Autodesk Inventor part; units mm, degrees
ref_plane "YZ Plane" through (0, 0, 0) normal (1, 0, 0) x (0, 1, 0)
ref_plane "XZ Plane" through (0, 0, 0) normal (0, 1, 0) x (-1, 0, 0)
ref_plane "XY Plane" through (0, 0, 0) normal (0, 0, 1) x (1, 0, 0)
sketch "Szkic1" plane through (0, 0, 0) normal (0, 0, 1) x (1, 0, 0)
  line L0 (-9.5177, 6.3249) -> (9.4823, 6.3249)
  line L1 (9.4823, 6.3249) -> (9.4823, -21.6751)
  line L2 (9.4823, -21.6751) -> (-9.5177, -21.6751)
  line L3 (-9.5177, -21.6751) -> (-9.5177, 6.3249)
  point P0 (0, 0)
  dimension "d0" = 19
  dimension "d1" = 28
extrude "Wyciągnięcie proste1" add sketch "Szkic1" along normal blind 12
chamfer "Faza1" distance 5 angle 45 2 edges at (9.4823, 6.3249, 6) (9.4823, -21.6751, 6)
fillet "Zaokrąglenie1" radius 4 2 edges at (-9.5177, 6.3249, 6) (-9.5177, -21.6751, 6)
sketch "Szkic2" plane through (0, 0, 0) normal (0, 0, -1) x (-1, 0, 0)
  line L0 (-4.4823, -21.6751) -> (5.5177, -21.6751)
  line L1 (5.5177, 6.3249) -> (-4.4823, 6.3249)
  arc A0 (5.5177, -21.6751) -> (9.5177, -17.6751) centre (5.5177, -17.6751) ccw
  line L2 (9.5177, -17.6751) -> (9.5177, 2.3249)
  arc A1 (9.5177, 2.3249) -> (5.5177, 6.3249) centre (5.5177, 2.3249) ccw
  line L3 (5.5177, 6.3249) -> (-4.4823, 6.3249)
  line L4 (-9.4823, 1.3249) -> (-4.4823, 6.3249)
  line L5 (-9.4823, 1.3249) -> (-9.4823, -16.6751)
  line L6 (-4.4823, -21.6751) -> (-9.4823, -16.6751)
  line L7 (-4.4823, -21.6751) -> (5.5177, -21.6751)
  line L8 (7.5177, 2.3249) -> (7.5177, -17.6751)
  arc A2 (5.5177, -19.6751) -> (7.5177, -17.6751) centre (5.5177, -17.6751) ccw
  line L9 (5.5177, -19.6751) -> (-3.6539, -19.6751)
  line L10 (-3.6539, -19.6751) -> (-7.4823, -15.8467)
  line L11 (-7.4823, -15.8467) -> (-7.4823, 0.4965)
  line L12 (-7.4823, 0.4965) -> (-3.6539, 4.3249)
  line L13 (-3.6539, 4.3249) -> (5.5177, 4.3249)
  arc A3 (7.5177, 2.3249) -> (5.5177, 4.3249) centre (5.5177, 2.3249) ccw
  line L14 (10.5177, 2.3249) -> (10.5177, -17.6751)
  line L15 (-10.4823, 2.3249) -> (-10.4823, -17.6751)
  circle A4 centre (0.5177, 11.8249) radius 2.5
  circle A5 centre (0.5177, -27.1751) radius 2.5
  line L16 (-10.4823, -17.6751) -> (-1.4174, -28.7579)
  line L17 (10.5177, 2.3249) -> (2.5396, 13.2953)
  line L18 (10.5177, -17.6751) -> (2.5396, -28.6455)
  line L19 (-10.4823, 2.3249) -> (-1.4174, 13.4077)
  point P0 (0, 0)
  dimension "d8" = 28
  dimension "d9" = 2
  dimension "d10" = 20
  dimension "d11" = 1
  dimension "d12" = 4
  dimension "d13" = 20
  dimension "d14" = 1
  dimension "d15" = 4
  dimension "d16" = 10
  dimension "d17" = 10
  dimension "d18" = 39
  dimension "d19" = 5.5
  dimension "d20" = 5
  dimension "d21" = 5
extrude "Wyciągnięcie proste2" add sketch "Szkic2" along normal blind 5.5 contours L6 L5 L4 L1 A1 L2 A0 L0 | L14 L18 A5 L16 L15 L19 A4 L17 | A4 | A5
extrude "Wyciągnięcie proste3" cut sketch "Szkic2" against normal blind 11 contours L8 A2 L9 L10 L11 L12 L13 A3
hole "Otwór1" at (-0.5177, 11.8249, 0) at (-0.5177, -27.1751, 0) direction (0, 0, -1) diameter 3 end through all
sketch "Szkic3" plane through (0, 0, -5.5) normal (0, 0, -1) x (-1, 0, 0)
  circle A0 centre (0.5177, 11.8249) radius 1.5
  circle A1 centre (0.5177, -27.1751) radius 1.5
  arc A2 (5.5177, -19.6751) -> (7.5177, -17.6751) centre (5.5177, -17.6751) ccw
  line L0 (5.5177, -19.6751) -> (-3.6539, -19.6751)
  line L1 (-3.6539, -19.6751) -> (-7.4823, -15.8467)
  line L2 (-7.4823, -15.8467) -> (-7.4823, 0.4965)
  line L3 (-7.4823, 0.4965) -> (-3.6539, 4.3249)
  line L4 (-3.6539, 4.3249) -> (5.5177, 4.3249)
  arc A3 (7.5177, 2.3249) -> (5.5177, 4.3249) centre (5.5177, 2.3249) ccw
  line L5 (7.5177, 2.3249) -> (7.5177, -17.6751)
  arc A4 (-1.4174, -28.7579) -> (2.5396, -28.6455) centre (0.5177, -27.1751) ccw
  line L6 (2.5396, -28.6455) -> (10.5177, -17.6751)
  line L7 (10.5177, -17.6751) -> (10.5177, 2.3249)
  line L8 (10.5177, 2.3249) -> (2.5396, 13.2953)
  arc A5 (2.5396, 13.2953) -> (-1.4174, 13.4077) centre (0.5177, 11.8249) ccw
  line L9 (-1.4174, 13.4077) -> (-10.4823, 2.3249)
  line L10 (-10.4823, 2.3249) -> (-10.4823, -17.6751)
  line L11 (-10.4823, -17.6751) -> (-1.4174, -28.7579)
  line L12 (6.5179, 7.8249) -> (-5.9837, 7.8249)
  line L13 (6.5179, -23.1751) -> (-5.9837, -23.1751)
  point P0 (0, 0)
  dimension "d33" = 31
  dimension "d34" = 39
  dimension "d35" = 4
extrude "Wyciągnięcie proste4" cut sketch "Szkic3" against normal blind 2 contours L11 L13 L6 A4 | L9 A5 L8 L12
fillet "Zaokrąglenie2" radius 1 4 edges at (-0.2671, 7.8249, -5.5) (-0.2671, 7.8249, -3.5) (-0.2671, -23.1751, -3.5) (-0.2671, -23.1751, -5.5)
fillet "Zaokrąglenie3" radius 5 4 edges at (-10.5177, 2.3249, -2.75) (-10.5177, -17.6751, -2.75) (10.4823, 2.3249, -2.75) (10.4823, -17.6751, -2.75)
sketch "Szkic4" plane through (0, 0, 11) normal (0, 0, -1) x (-1, 0, 0)
  line L0 (7.5177, 2.3249) -> (7.5177, -17.6751)
  arc A0 (7.5177, 2.3249) -> (5.5177, 4.3249) centre (5.5177, 2.3249) ccw
  line L1 (-3.6539, 4.3249) -> (5.5177, 4.3249)
  line L2 (-7.4823, 0.4965) -> (-3.6539, 4.3249)
  line L3 (-7.4823, -15.8467) -> (-7.4823, 0.4965)
  line L4 (-3.6539, -19.6751) -> (-7.4823, -15.8467)
  line L5 (5.5177, -19.6751) -> (-3.6539, -19.6751)
  arc A1 (5.5177, -19.6751) -> (7.5177, -17.6751) centre (5.5177, -17.6751) ccw
  line L6 (4.5177, 0.8249) -> (0.5177, 0.8249)
  line L7 (0.5177, 0.8249) -> (0.5177, -1.1751)
  line L8 (0.5177, -1.1751) -> (4.5177, -1.1751)
  line L9 (4.5177, -1.1751) -> (4.5177, 0.8249)
  line L10 (4.5177, -14.1751) -> (0.5177, -14.1751)
  line L11 (0.5177, -14.1751) -> (0.5177, -16.1751)
  line L12 (0.5177, -16.1751) -> (4.5177, -16.1751)
  line L13 (4.5177, -16.1751) -> (4.5177, -14.1751)
  line L14 (-1.4823, -6.6751) -> (-5.4823, -6.6751)
  line L15 (-5.4823, -6.6751) -> (-5.4823, -8.6751)
  line L16 (-5.4823, -8.6751) -> (-1.4823, -8.6751)
  line L17 (-1.4823, -8.6751) -> (-1.4823, -6.6751)
  point P0 (0, 0)
  dimension "d40" = 4
  dimension "d41" = 2
  dimension "d42" = 4
  dimension "d43" = 2
  dimension "d44" = 4
  dimension "d45" = 2
  dimension "d46" = 13
  dimension "d47" = 24
  dimension "d48" = 3.5
  dimension "d49" = 5.5
  dimension "d50" = 2
  dimension "d51" = 3
  dimension "d52" = 3
extrude "Wyciągnięcie proste5" add sketch "Szkic4" along normal blind 15 contours L9 L8 L7 L6 | L13 L12 L11 L10 | L17 L16 L15 L14
fillet "Zaokrąglenie4" radius 2 6 edges at (1.4823, -7.6751, -4) (5.4823, -7.6751, -4) (-0.5177, -0.1751, -4) (-4.5177, -0.1751, -4) (-0.5177, -15.1751, -4) (-4.5177, -15.1751, -4)
sketch "Szkic5" plane through (0, 0, 12) normal (0, 0, 1) x (1, 0, 0)
  arc A0 (-9.5177, -17.6751) -> (-5.5177, -21.6751) centre (-5.5177, -17.6751) ccw
  line L0 (-5.5177, -21.6751) -> (4.4823, -21.6751)
  line L1 (9.4823, -16.6751) -> (4.4823, -21.6751)
  line L2 (9.4823, -16.6751) -> (9.4823, 1.3249)
  line L3 (4.4823, 6.3249) -> (9.4823, 1.3249)
  line L4 (4.4823, 6.3249) -> (-5.5177, 6.3249)
  arc A1 (-5.5177, 6.3249) -> (-9.5177, 2.3249) centre (-5.5177, 2.3249) ccw
  line L5 (-9.5177, 2.3249) -> (-9.5177, -17.6751)
  line L6 (-0.5177, -14.1751) -> (-4.5177, -14.1751)
  line L7 (-4.5177, -16.1751) -> (-0.5177, -16.1751)
  line L8 (-4.5177, -14.1751) -> (-4.5177, -16.1751)
  line L9 (-0.5177, -16.1751) -> (-0.5177, -14.1751)
  line L10 (-4.5177, -1.1751) -> (-0.5177, -1.1751)
  line L11 (-0.5177, 0.8249) -> (-4.5177, 0.8249)
  line L12 (-4.5177, 0.8249) -> (-4.5177, -1.1751)
  line L13 (-0.5177, -1.1751) -> (-0.5177, 0.8249)
  line L14 (1.4823, -8.6751) -> (5.4823, -8.6751)
  line L15 (5.4823, -6.6751) -> (1.4823, -6.6751)
  line L16 (5.4823, -8.6751) -> (5.4823, -6.6751)
  line L17 (1.4823, -6.6751) -> (1.4823, -8.6751)
  line L18 (-5.5177, -17.1751) -> (0.4823, -17.1751)
  line L19 (0.4823, -17.1751) -> (0.4823, -13.1751)
  line L20 (0.4823, -13.1751) -> (-5.5177, -13.1751)
  line L21 (-5.5177, -13.1751) -> (-5.5177, -17.1751)
  line L22 (0.4823, -9.6751) -> (6.4823, -9.6751)
  line L23 (6.4823, -9.6751) -> (6.4823, -5.6751)
  line L24 (6.4823, -5.6751) -> (0.4823, -5.6751)
  line L25 (0.4823, -5.6751) -> (0.4823, -9.6751)
  line L26 (0.4823, 1.8249) -> (-5.5177, 1.8249)
  line L27 (-5.5177, 1.8249) -> (-5.5177, -2.1751)
  line L28 (-5.5177, -2.1751) -> (0.4823, -2.1751)
  line L29 (0.4823, -2.1751) -> (0.4823, 1.8249)
  point P0 (0, 0)
  dimension "d56" = 1
  dimension "d57" = 1
  dimension "d58" = 1
extrude "Wyciągnięcie proste6" add sketch "Szkic5" along normal blind 10 contours L9 L7 L8 L6 | L12 L11 L13 L10 | L17 L15 L16 L14
extrude "Wyciągnięcie proste7" add sketch "Szkic5" along normal blind 4 contours L21 L20 L19 L18 | L25 L24 L23 L22 | L29 L28 L27 L26
fillet "Zaokrąglenie5" radius 1 6 edges at (-4.5177, -15.1751, 22) (-0.5177, -15.1751, 22) (-4.5177, -0.1751, 22) (-0.5177, -0.1751, 22) (1.4823, -7.6751, 22) (5.4823, -7.6751, 22)
equation "\"d12\" = -0.5 * d10 + 0.5 * d8"
equation "\"d14\" = d11"
equation "\"d15\" = d12"
equation "\"d35\" = -0.5 * d33 + 0.5 * d34"
properties part number "COTS_GENERIC_AC_Power_Socket_C14"
Model file for the job. Use its own axes, mm. A direction names the side the tool comes from. Round coordinates to 2 decimals unless told otherwise and drop trailing zeros. Loops run counter-clockwise (first coordinate to the right, second up) from the corner with the lowest first, then second, coordinate; pieces in that order, holes last. Notation, with made-up numbers: M -1.75,61 L 47.25,61 A22 ccw 47.25,98 Z; hole C -9,-3 d10. An arc over 180 degrees is marked long. Put each result on its own line as item: value. Start each with the question number.
Item 1: Drill centre lines: line 1 along Y through (x, z) = (2.25, 4); line 2 along Y through (x, z) = (-3.5, 19); line 3 along X through (y, z) = (-8, 10.5). Where is each one in solid material? Low to high.
Item 2: Cut at C-C (z = -0.75). Give the number of separate pieces and of enclosed holes in the cut face, then the cut area to 3 significant figures.
Item 3: Cut at B-B (y = -3.5). List the corners of the cut face in (x, z).
Item 4: Drop flat-ended pins along their axis: P1, Ø12, axis at x = 2.5, z = 12.5, coming from the -Y side; P2, Ø3, axis at x = 5, y = -18, coming from the +Z side; P3, Ø2, axis at y = -15, z = 6.5, coming from the +X side. Give the stop position or say it passes through.
Item 5: Cut at D-D (z = 12.75). List the corners of the cut face in (x, y), then the cut area to 3 significant figures.
Item 6: Cut at A-A (z = 7). List the corners of the cut face in (x, y), then the cut area to 3 significant figures.
Item 7: Mould opens along X. For faces 1 (the face through (-0.12, -22.89, -5.2)), 2 (the face through (-0.557, 14.325, -1.726)), 3 (the face through (-1, 4.325, 3)) say: released by +X, released by -X, zero draft, split by the parting line, or undercut.
Item 8: 3-axis set-ups, long thin cutter, end or side, ignore diameter. For faces 4 (the face through (-2, -13.175, 14)), 5 (the face through (-5.518, 0, 14)), 6 (the face through (5.482, -8, 5)), 7 (the face through (0, 10, -3.5)): which of +Z, -Z, +X, -X, +Y, -Y reach the whole face in a straight line?
Answer block:
1. line 1: -21.68 to -19.68, -8.68 to -6.68, 4.32 to 6.32
1. line 2: -16.18 to -14.18, -1.18 to 0.82
1. line 3: -9.52 to -7.52, 1.48 to 5.48, 7.48 to 9.48
2. separate pieces: 4
2. enclosed holes: 3
2. area: 366 mm2
3. outline: M -10.52,-5.5 L -7.52,-5.5 L -7.52,11 L 7.48,11 L 7.48,-5.5 L 10.48,-5.5 L 10.48,0 L 9.48,0 L 9.48,12 L -9.52,12 L -9.52,0 L -10.52,0 Z
4. P1: y = -21.68
4. P2: z = 12
4. P3: x = 9.48
5. outline: M -5.52,-17.18 L 0.48,-17.18 L 0.48,-13.18 L -5.52,-13.18 Z; M -5.52,-2.18 L 0.48,-2.18 L 0.48,1.82 L -5.52,1.82 Z; M 0.48,-9.68 L 6.48,-9.68 L 6.48,-5.68 L 0.48,-5.68 Z
5. area: 72.0 mm2
6. outline: M -9.52,-17.68 A4 ccw -5.52,-21.68 L 4.48,-21.68 L 9.48,-16.68 L 9.48,1.32 L 4.48,6.32 L -5.52,6.32 A4 ccw -9.52,2.32 Z; M -4.52,-16.18 L -0.52,-16.18 L -0.52,-14.18 L -4.52,-14.18 Z; M -4.52,-1.18 L -0.52,-1.18 L -0.52,0.82 L -4.52,0.82 Z; M 1.48,-8.68 L 5.48,-8.68 L 5.48,-6.68 L 1.48,-6.68 Z; hole M -7.52,-17.68 A2 ccw -5.52,-19.68 L 3.65,-19.68 L 7.48,-15.85 L 7.48,0.5 L 3.65,4.32 L -5.52,4.32 A2 ccw -7.52,2.32 Z
6. area: 181 mm2
7. face 1: zero draft
7. face 2: split by the parting line
7. face 3: undercut
8. face 4: +Z, +X, -X
8. face 5: +Z, -X, +Y, -Y
8. face 6: -Z
8. face 7: -Z, +X, -X, +Y
